from build123d import *

# Parameters (mm, degrees)
F1_DEPTH      = 2.5
F1_DEPTH_BACK = 2.5
F3_R          = 1.5
F4_DEPTH      = 5.001
F6_DEPTH      = 2
F7_R          = 2


with BuildPart() as f1:
    # F0 (on Front) → F1 (new body, two sides)
    with BuildSketch(Plane.XZ) as f1_sk:
        Polygon((-3.7, 0), (0, 0), (3.7, 0), (5, 1.3), (5, 3), (2.75, 3), (2.75, 5), (0, 5), (-2.75, 5), (-2.75, 3), (-5, 3), (-5, 1.3), align=None)
    extrude(amount=F1_DEPTH)
    extrude(f1_sk.sketch, amount=-F1_DEPTH_BACK)

    # F3 (on face) → F4 (cut, through all)
    with BuildSketch(Plane.XY.offset(5)):
        Circle(F3_R)
    extrude(amount=-F4_DEPTH, mode=Mode.SUBTRACT)

    # F5 (on face) → F6 (cut, through all)
    with BuildSketch(Plane.XY.offset(5)):
        with BuildLine():
            Line((2.75, -2.5), (2.75, 0))
            ThreePointArc((2.75, 0), (2.314413618, -1.4852574204), (1.1456439237, -2.5))
            Line((1.1456439237, -2.5), (2.75, -2.5))
        make_face()
        with BuildLine():
            ThreePointArc((-2.75, 0), (-2.314413618, 1.4852574204), (-1.1456439237, 2.5))
            Line((-1.1456439237, 2.5), (-2.75, 2.5))
            Line((-2.75, 2.5), (-2.75, 0))
        make_face()
    extrude(amount=-F6_DEPTH, mode=Mode.SUBTRACT)

    # F7
    f7_edges = [f1.edges().sort_by_distance(p)[0] for p in [
        (5, -2.5, 2.15),
        (-5, 2.5, 2.15),
    ]]
    fillet(f7_edges, radius=F7_R)


solid = f1.part
The model under review builds one solid part; all positions refer to its coordinate system, in mm. A direction names the side the tool comes from. Give positions to 0.01 mm unless a question says otherwise; leave off trailing zeros. Order: outer loops, then holes, each group sorted by start corner. A loop starts at its lowest first (then second) coordinate and runs counter-clockwise, first axis right, second up. Notation, with made-up numbers: M 85,3.5 L 126,3.5 A32 cw 126,31.5 Z; hole C 20.5,-19.5 d9. An arc over 180 degrees is marked long. Use one line per item in the form item = value. Start each with the question number.
Item 1: Insertion check: pin 1 Ø1.2 at (x, y) = (-3.5, 1) entering from +Z; pin 2 Ø0.6 at (y, z) = (-1, 4.5) entering from -X; pin 3 Ø2.5 at (x, y) = (0, 0) entering from +Z; pin 4 Ø0.6 at (y, z) = (0.5, 4) entering from +X. Each pin has a flat end and moves straight along its axis. Give the tip position at first contact, or say it passes through.
Item 2: To check wall thickness, follow line 1 along Y through (x, z) = (0, 3); line 2 along Z through (x, y) = (-3.5, 0.15); line 3 along Y through (x, z) = (-2.5, 4.1). State the ranges of each line that lie inside material, in increasing order. Write a range as from..to.
Item 3: The part is to be moulded in two halves that separate along Y. For faces 1 (the cylindrical face through (-1.5, 0.07, 2.54)), 2 (the cylindrical face through (-4.2, 2.1, 1.8)), 3 (the flat face through (-4, 0, 3)), 4 (the cylindrical face through (4.2, -2.1, 1.9)), say which applies: pulls with the +Y half, pulls with the -Y half, needs draft (parallel to the pull), parting line crosses it, or undercut.
Item 4: For faces 5 (the cylindrical face through (2.326, -1.467, 4.014)), 6 (the flat face through (2.75, 1, 4)), 7 (the flat face through (-2.75, -1, 4)), list the 3-axis set-ups (+Z, -Z, +X, -X, +Y, -Y) from which the entire face can be reached by the end or side of a thin tool; tool diameter is ignored.
Item 5: We need section C-C on y = 1.2. Give the boundary of the cut face in (x, z).
Item 6: We need section A-A on x = 0. Give the boundary of the cut face in (y, z).
Item 7: We need section B-B on z = 2.3. Give the boundary of the cut face in (x, y), plus the area to 3 significant figures.
Item 8: We need section D-D on z = 3.7. Give the boundary of the cut face in (x, y), plus the area to 3 significant figures.
Completed:
q1.pin_1 = 3
q1.pin_2 = -2.75
q1.pin_3 = through
q1.pin_4 = 2.75
q2.line_1 = -2.5..-1.5, 1.5..2.5
q2.line_2 = 0..3
q2.line_3 = -2.5..1.15
q3.face_1 = undercut
q3.face_2 = pulls with the +Y half
q3.face_3 = needs draft
q3.face_4 = pulls with the -Y half
q4.face_5 = +Z, +X, -Y
q4.face_6 = +Z, +X, +Y, -Y
q4.face_7 = +Z, -X, +Y, -Y
q5.outline = M -4.87,1.17 L -3.7,0 L -0.9,0 L -0.9,5 L -2.47,5 L -2.47,3 L -4.87,3 Z; M 0.9,0 L 3.7,0 L 5,1.3 L 5,3 L 2.75,3 L 2.75,5 L 0.9,5 Z
q6.outline = M -2.5,0 L -1.5,0 L -1.5,5 L -2.5,5 Z; M 1.5,0 L 2.5,0 L 2.5,5 L 1.5,5 Z
q7.outline = M -5,-2.5 L 3,-2.5 A2 ccw 5,-0.5 L 5,2.5 L -3,2.5 A2 ccw -5,0.5 Z; hole C 0,0 d3
q7.area = 41.2 mm²
q8.outline = M -2.75,-2.5 L 1.15,-2.5 A2.75 ccw 2.75,0 L 2.75,2.5 L -1.15,2.5 A2.75 ccw -2.75,0 Z; hole C 0,0 d3
q8.area = 18.2 mm²
